The model under review builds one solid part; all positions refer to its coordinate system, in mm. Face numbers are marked on the shaded views. A direction names the side the tool comes from. Coordinates: 2 decimals unless noted, no trailing zeros. Order: outer loops, then holes, each group sorted by start corner. A loop starts at its lowest first (then second) coordinate and runs counter-clockwise, first axis right, second up. Notation, with made-up numbers: (11, -14.5) - (42, -14.5) arc R29 cw to (42, 10.5) - close; hole circle Ø8 at (49, 53.5). An arc over 180 degrees is marked (long way). Answer in a Markdown table with one row per item.
```python
from build123d import *

# Parameters (mm, degrees)
PAD_DEPTH       = 15
SKETCH001_R     = 2.5
POCKET_DEPTH    = 6
SKETCH002_R     = 2.486179
SKETCH002_R_2   = 2.528636
POCKET001_DEPTH = 6


with BuildPart() as part:
    # Sketch → Pad (new body)
    with BuildSketch(Plane.YZ):
        Polygon((-126.2253788048, 0), (0, 0), (0, 5), (-7.0710678119, 12.0710678119), (-11.1015764646, 8.0405591591), (-81.8122545833, 78.7512372778), (-77.7817459305, 82.7817459305), (-90.5096679919, 95.5096679919), (-102.7772339365, 95.5096679919), (-126.2253788048, 8), align=None)
        with BuildLine():
            Line((-93.9680126151, 79.5932868106), (-27.8685100548, 13.4937842503))
            ThreePointArc((-30.14411, 8), (-27.1708953887, 9.9866384892), (-27.8685100548, 13.4937842503))
            Line((-30.14411, 8), (-112.060173, 8))
            ThreePointArc((-116.4205378609, 13.6825381216), (-115.6415142719, 9.7661220673), (-112.060173, 8))
            Line((-116.4205378609, 13.6825381216), (-99.1304524836, 78.2100152169))
            ThreePointArc((-93.9680126151, 79.5932868106), (-96.9485486629, 80.3919190376), (-99.1304524836, 78.2100152169))
        make_face(mode=Mode.SUBTRACT)
    extrude(amount=PAD_DEPTH)

    # Sketch001 (on Face8 of Pad) → Pocket (cut)
    with BuildSketch(Plane(origin=(0, 2.5, 2.5), x_dir=(0, -0.7071067812, 0.7071067812), z_dir=(0, 0.7071067812, 0.7071067812))):
        with Locations((8.5355339059, 7.6199603564)):
            Circle(SKETCH001_R)
        with Locations((124.5355339037, 7.6192468054)):
            Circle(SKETCH001_R)
    extrude(amount=-POCKET_DEPTH, mode=Mode.SUBTRACT)

    # Cone → Cone (revolve)
    with BuildSketch(Plane(origin=(7.5, -123.3933483575, 18.569281518), x_dir=(0, -0.2588190451, -0.9659258263), z_dir=(-1, 0, 0))):
        Polygon((0, 0), (6.5, 0), (3.5, 3), (0, 3), align=None)
    revolve(axis=Axis((7.5, -123.3933483575, 18.569281518), (0, -0.9659258263, 0.2588190451)))

    # Cone001 → Cone001 (revolve)
    with BuildSketch(Plane(origin=(7.5, -110.7112151475, 65.8996470062), x_dir=(0, -0.2588190451, -0.9659258263), z_dir=(-1, 0, 0))):
        Polygon((0, 0), (6.5, 0), (3.5, 3), (0, 3), align=None)
    revolve(axis=Axis((7.5, -110.7112151475, 65.8996470062), (0, -0.9659258263, 0.2588190451)))

    # Sketch002 (on Face21 of Cone001) → Pocket001 (cut)
    with BuildSketch(Plane(origin=(7.5, -113.6089926263, 66.6761041415), x_dir=(0, -0.2588190451, -0.9659258263), z_dir=(0, -0.9659258263, 0.2588190451))):
        Circle(SKETCH002_R)
        with Locations((48.9999960198, -0.01975)):
            Circle(SKETCH002_R_2)
    extrude(amount=-POCKET001_DEPTH, mode=Mode.SUBTRACT)


solid = part.part
```
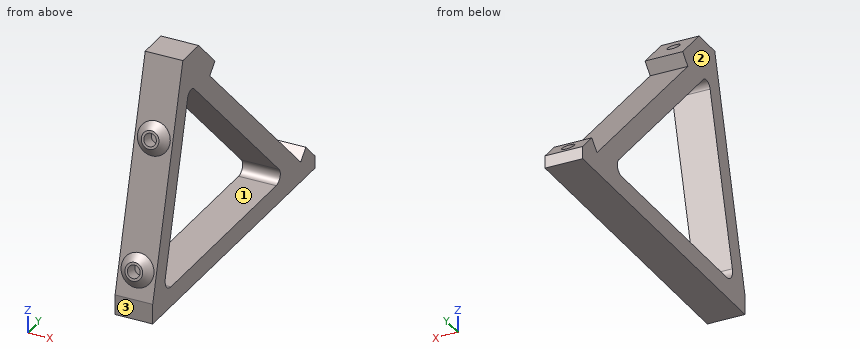
Item 1: We need section D-D, the plane y = -23. Write out the cut boundary in (x, z).
Check values:
| item | result |
|---|---|
| outline | (0, 0) - (15, 0) - (15, 19.94) - (0, 19.94) - close |
Item 2: Clearance check with flat-ended pins moving along their axes: pin 1 Ø2 at (y, z) = (-89.5, 10.5) entering from -X; pin 2 Ø1.5 at (x, y) = (9.5, -88) entering from +Z; pin 3 Ø6.5 at (x, z) = (4, 2.5) entering from -Y; pin 4 Ø5 at (x, z) = (8.5, 36.5) entering from -Y. State where each tip first meets the part, or that it passes through.
Check values:
| item | result |
|---|---|
| pin 1 | through |
| pin 2 | z = 93.75 |
| pin 3 | y = -126.23 |
| pin 4 | y = -119.26 |
Item 3: We need section C-C, the plane y = -79.5. Write out the cut boundary in (x, z).
Check values:
| item | result |
|---|---|
| outline | (0, 0) - (15, 0) - (15, 8) - (0, 8) - close; (0, 65.13) - (15, 65.13) - (15, 76.44) - (0, 76.44) - close; (0, 81.06) - (15, 81.06) - (15, 84.5) - (0, 84.5) - close |
Item 4: We need section B-B, the plane y = -61.5. Write out the cut boundary in (x, z).
Check values:
| item | result |
|---|---|
| outline | (0, 0) - (15, 0) - (15, 8) - (0, 8) - close; (0, 47.13) - (15, 47.13) - (15, 58.44) - (0, 58.44) - close |
Item 5: We need section A-A, the plane z = 34. Write out the cut boundary in (x, y), then the cut area to 3 significant figures.
Check values:
| item | result |
|---|---|
| outline | (0, -119.26) - (15, -119.26) - (15, -110.98) - (0, -110.98) - close; (0, -48.37) - (15, -48.37) - (15, -37.06) - (0, -37.06) - close |
| area | 294 mm^2 |
Item 6: Tool access review of the marked faces 1, 2 and 3: name each direction out of +Z, -Z, +X, -X, +Y, -Y from which nothing blocks a thin tool from reaching the whole face with its end or side.
Check values:
| item | result |
|---|---|
| face 1 | +X, -X |
| face 2 | +Z, -Z, -X, +Y, -Y |
| face 3 | -Z, +X, -X, -Y |
Item 7: To check wall thickness, follow line 1 (Z direction, x = 6, y = -80.5); line 2 (Z direction, x = 14.75, y = -78); line 3 (Y direction, x = 13.25, z = 72). State the ranges of each line that lie inside material, in increasing order. Write a range as from..to.
Check values:
| item | result |
|---|---|
| line 1 | 0..8, 66.13..77.44, 80.06..85.5 |
| line 2 | 0..8, 63.63..74.94, 82.56..83 |
| line 3 | -109.08..-100.79, -86.37..-75.06 |
